Check sheet for the drawn part. Datum: minimum x, y, z corner. Units: mm. Give positions to 0.01 mm unless a question says otherwise; leave off trailing zeros. Order: outer loops, then holes, each group sorted by start corner. A loop starts at its lowest first (then second) coordinate and runs counter-clockwise, first axis right, second up.
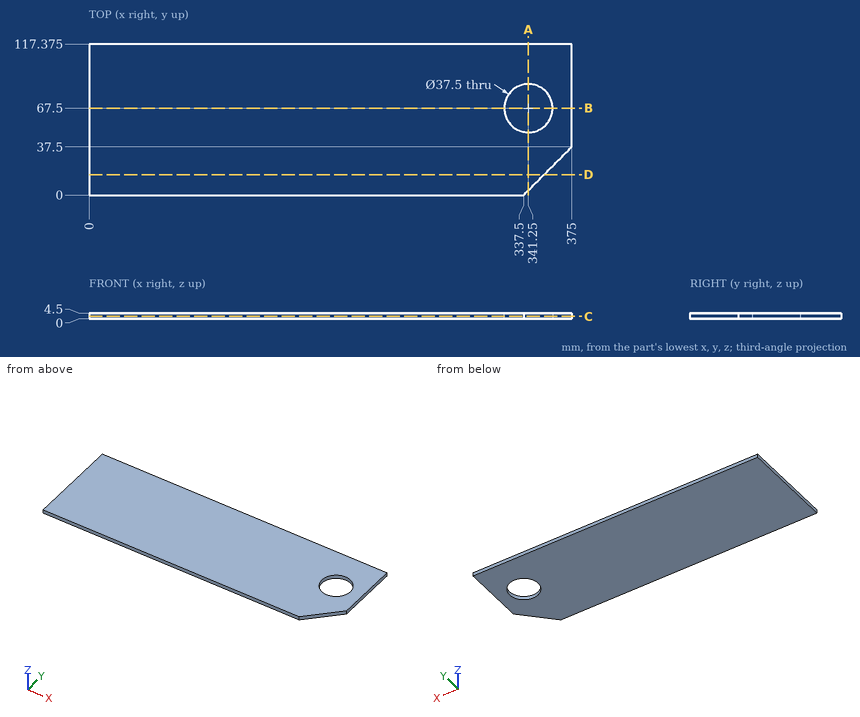
(1) Section check B-B, the plane y = 67.5. Enter the section's corners in (x, z), then the cut area to 3 significant figures.
Solved:
outline: (0, 0) - (322.5, 0) - (322.5, 4.5) - (0, 4.5) - close; (360, 0) - (375, 0) - (375, 4.5) - (360, 4.5) - close
area: 1,520 mm2
(2) Section check C-C, the plane z = 1.95. Enter the section's corners in (x, y) (3 decimals).
Solved:
outline: (0, 0) - (337.5, 0) - (375, 37.5) - (375, 117.375) - (0, 117.375) - close; hole circle Ø37.5 at (341.25, 67.5)
(3) Scan lines: line 1 (Y direction, x = 341.25, z = 3.5) (3 decimals); line 2 (Y direction, x = 336, z = 2.2) (3 decimals); line 3 (X direction, y = 52, z = 0.65). Record each from-to range of solid material in increasing order.
Solved:
line 1: y = 3.75 to 48.75, 86.25 to 117.375
line 2: y = 0 to 49.5, 85.5 to 117.375
line 3: x = 0 to 330.7, 351.8 to 375
(4) Section check A-A, the plane x = 341.25. Enter the section's corners in (y, z) (3 decimals), then the cut area to 3 significant figures.
Solved:
outline: (3.75, 0) - (48.75, 0) - (48.75, 4.5) - (3.75, 4.5) - close; (86.25, 0) - (117.375, 0) - (117.375, 4.5) - (86.25, 4.5) - close
area: 343 mm2
(5) Section check D-D, the plane y = 16. Enter the section's corners in (x, z).
Solved:
outline: (0, 0) - (353.5, 0) - (353.5, 4.5) - (0, 4.5) - close
